Work out the finished part from the listing and answer in its coordinate system (mm). Round coordinates to 2 decimals unless told otherwise and drop trailing zeros.
1. Straight lines are drawn through the part: probe 1 along Y at (x, z) = (12.5, 0.45); probe 2 along Y at (x, z) = (47.5, 0.2). For each, find the intervals that lie inside material, in ascending order.
2. Determine the mould class of faces 1 (the face through (32, 15, 0)), 2 (the face through (64.14, 29.1, 0.51)), 3 (the face through (62.79, 25.96, 0.51)), 4 (the face through (0.86, 0.9, 0.51)) for opening direction X: pulls with the +X half, pulls with the -X half, needs draft (parallel to the pull), parting line crosses it, or undercut.
3. Find section A-A (z = 0.8). Count the separate pieces of the cut face and the enclosed holes in it, and give its area (3 significant figures).
4. A flat-ended cylindrical pin translates along its axis: pin 1 Ø2 at (x, y) = (61.5, 26.5) entering from -Z. Find the tip coordinate at first contact, or state that the pin passes through.
```python
from build123d import *

# Parameters (mm, degrees)
SKETCH_W                        = 65
SKETCH_H                        = 30
PAD_DEPTH                       = 1
FILLET_R                        = 3
SKETCH001_R                     = 1.4
POCKET_DEPTH                    = 5
LINEARPATTERN_COUNT             = 2
LINEARPATTERN_PITCH             = 58
LINEARPATTERN001_COUNT          = 2
LINEARPATTERN001_PITCH          = 23
SKETCH001_LINEARPATTERN002_2_R  = 1.4
POCKET_LINEARPATTERN002_2_DEPTH = 5
LINEARPATTERN003_COUNT          = 2
LINEARPATTERN003_PITCH          = 23
SKETCH003_R                     = 0.5
POCKET001_DEPTH                 = 5
LINEARPATTERN004_COUNT          = 20
LINEARPATTERN004_PITCH          = 2.673684


with BuildPart() as part:
    # Sketch → Pad (new body)
    with BuildSketch(Plane.XY):
        with Locations((32.5, 15)):
            Rectangle(SKETCH_W, SKETCH_H)
    extrude(amount=PAD_DEPTH)

    # Fillet
    fillet_edges = [part.edges().sort_by_distance(p)[0] for p in [
        (0, 0, 0.5),
        (65, 30, 0.5),
        (0, 30, 0.5),
        (65, 0, 0.5),
    ]]
    fillet(fillet_edges, radius=FILLET_R)

    # Sketch001 (on Face5 of Fillet) → Pocket (cut)
    with BuildSketch(Plane.XY.offset(1)):
        with Locations((3.5, 3.5)):
            Circle(SKETCH001_R)
    pocket = extrude(amount=-POCKET_DEPTH, mode=Mode.SUBTRACT)

    # LinearPattern: Pocket ×2
    with Locations(*[(i * LINEARPATTERN_PITCH, 0, 0) for i in range(1, LINEARPATTERN_COUNT)]):
        add(pocket, mode=Mode.SUBTRACT)

    # LinearPattern001: Pocket ×2
    with Locations(*[(0, i * LINEARPATTERN001_PITCH, 0) for i in range(1, LINEARPATTERN001_COUNT)]):
        add(pocket, mode=Mode.SUBTRACT)

    # Sketch001 LinearPattern002 2 → Pocket LinearPattern002 2 (cut)
    with BuildSketch(Plane(origin=(58, 0, 1), x_dir=(1, 0, 0), z_dir=(0, 0, 1))):
        with Locations((3.5, 3.5)):
            Circle(SKETCH001_LINEARPATTERN002_2_R)
    pocket_linearpattern002_2 = extrude(amount=-POCKET_LINEARPATTERN002_2_DEPTH, mode=Mode.SUBTRACT)

    # LinearPattern003: Pocket, Pocket LinearPattern002 2 ×2
    with Locations(*[(0, i * LINEARPATTERN003_PITCH, 0) for i in range(1, LINEARPATTERN003_COUNT)]):
        add(pocket, mode=Mode.SUBTRACT)
        add(pocket_linearpattern002_2, mode=Mode.SUBTRACT)

    # Sketch003 (on Face5 of MultiTransform) → Pocket001 (cut)
    with BuildSketch(Plane.XY.offset(1)):
        with Locations((7.1, 27.77)):
            Circle(SKETCH003_R)
        with Locations((7.1, 25.23)):
            Circle(SKETCH003_R)
    pocket001 = extrude(amount=-POCKET001_DEPTH, mode=Mode.SUBTRACT)

    # LinearPattern004: Pocket001 ×20
    with Locations(*[(i * LINEARPATTERN004_PITCH, 0, 0) for i in range(1, LINEARPATTERN004_COUNT)]):
        add(pocket001, mode=Mode.SUBTRACT)


solid = part.part
```
Worked answers:
1. probe 1: y = 0 to 24.73, 25.73 to 27.27, 28.27 to 30
1. probe 2: y = 0 to 24.83, 25.63 to 27.37, 28.17 to 30
2. face 1: needs draft
2. face 2: pulls with the +X half
2. face 3: undercut
2. face 4: pulls with the -X half
3. separate pieces: 1
3. enclosed holes: 44
3. area: 1,890 mm2
4. pin 1: passes through
